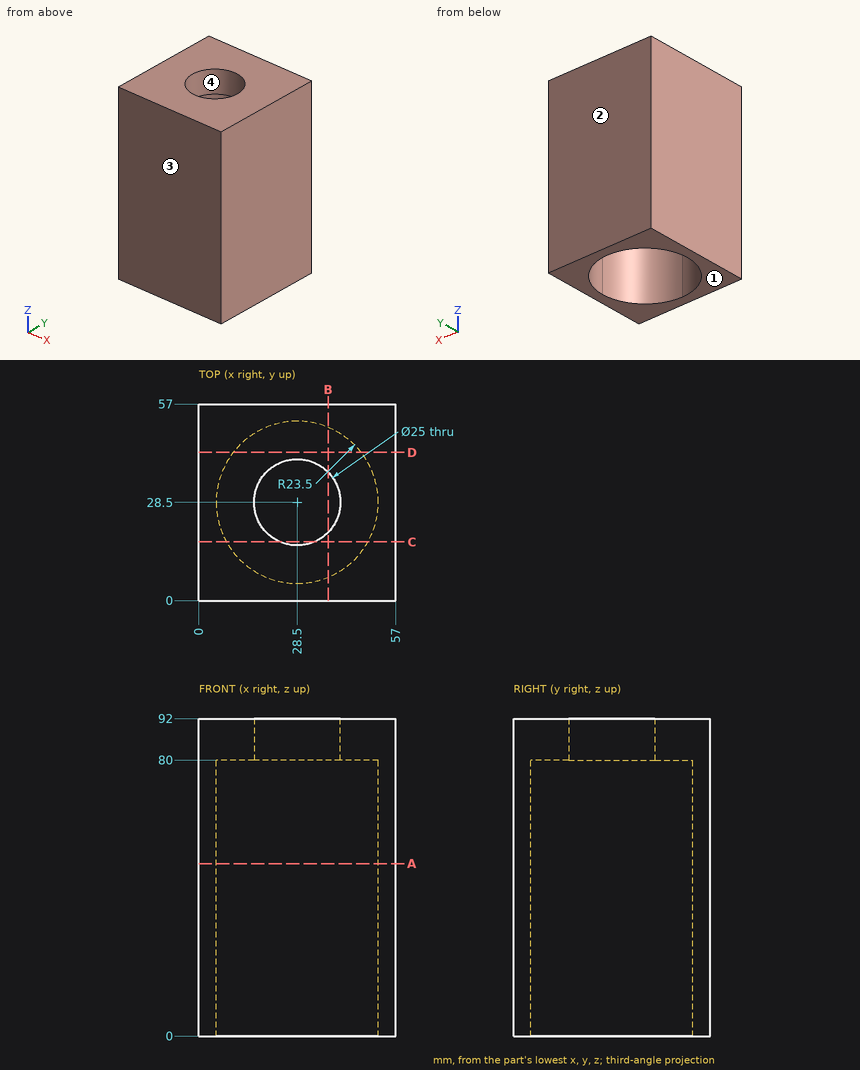
The drawing under review shows one solid part. Ordinate dimensions are in mm from its lowest x, y, z. Coordinates: 2 decimals unless noted, no trailing zeros. Order: outer loops, then holes, each group sorted by start corner. A loop starts at its lowest first (then second) coordinate and runs counter-clockwise, first axis right, second up. Notation, with made-up numbers: M 12,-27 L 43,-27 A38 cw 43,11 Z; hole C 53,49.5 d8. An arc over 180 degrees is marked long. Use a Markdown table: item, result.
(1) Add section C-C (y = 17). Give the boundary of the cut face in (x, z).
Worked answers:
| item | result |
|---|---|
| outline | M 0,0 L 8.01,0 L 8.01,80 L 23.6,80 L 23.6,92 L 0,92 Z; M 33.4,80 L 48.99,80 L 48.99,0 L 57,0 L 57,92 L 33.4,92 Z |
(2) Add section A-A (z = 50). Give the boundary of the cut face in (x, y).
Worked answers:
| item | result |
|---|---|
| outline | M 0,0 L 57,0 L 57,57 L 0,57 Z; hole M 5,28.5 A23.5 ccw 28.5,5 A23.5 ccw 52,28.5 A23.5 ccw 28.5,52 A23.5 ccw Z |
(3) Wall thickness on probe 1 along Y at (x, z) = (28, 88); probe 2 along X at (y, z) = (28.5, 85); probe 3 along Z at (x, y) = (26.5, 12): over which ranges is each line inside the solid? List them lowest first.
Worked answers:
| item | result |
|---|---|
| probe 1 | y = 0 to 16.01, 40.99 to 57 |
| probe 2 | x = 0 to 16, 41 to 57 |
| probe 3 | z = 80 to 92 |
(4) Draft analysis for pull direction Y (two halves, no side actions). For the marked faces 1, 2, 3 and 4, state which applies: released by +Y, released by -Y, zero draft, split by the parting line, or undercut.
Worked answers:
| item | result |
|---|---|
| face 1 | zero draft |
| face 2 | released by +Y |
| face 3 | released by -Y |
| face 4 | undercut |
(5) For P1, Ø10, axis at y = 24, z = 11, coming from the -X side; P2, Ø15, axis at x = 28.5, y = 28.5, coming from the +Z side; P3, Ø2, axis at x = 8, y = 26, coming from the -Z side, all flat-tipped, find the tip position at first contact; note any pin that passes through.
Worked answers:
| item | result |
|---|---|
| P1 | stops at x = 0 |
| P2 | passes through |
| P3 | stops at z = 80 |
(6) Add section D-D (y = 43). Give the boundary of the cut face in (x, z).
Worked answers:
| item | result |
|---|---|
| outline | M 0,0 L 10.01,0 L 10.01,80 L 46.99,80 L 46.99,0 L 57,0 L 57,92 L 0,92 Z |
(7) Add section B-B (x = 37.5). Give the boundary of the cut face in (y, z).
Worked answers:
| item | result |
|---|---|
| outline | M 0,0 L 6.79,0 L 6.79,80 L 19.83,80 L 19.83,92 L 0,92 Z; M 37.17,80 L 50.21,80 L 50.21,0 L 57,0 L 57,92 L 37.17,92 Z |
